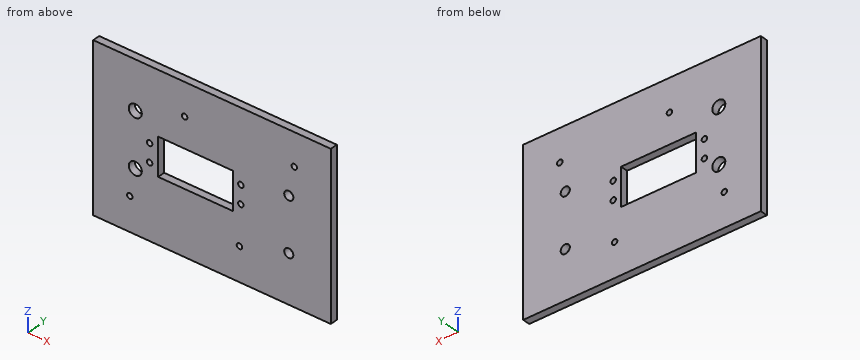
from build123d import *

# Parameters (mm, degrees)
SKETCH1_W           = 130
SKETCH1_H           = 90
BOSS_EXTRUDE1_DEPTH = 4
SKETCH7_R           = 3.65
SKETCH7_R_2         = 3.57
CUT_EXTRUDE5_DEPTH  = 10
SKETCH15_W          = 40.9
SKETCH15_H          = 20.7
CUT_EXTRUDE10_DEPTH = 5
SKETCH6_R           = 1.5
CUT_EXTRUDE4_DEPTH  = 4
SKETCH12_R          = 1.5
CUT_EXTRUDE8_DEPTH  = 5
SKETCH14_W          = 15.685038152
SKETCH14_H          = 44.965808151
SKETCH14_R          = 2.5
BOSS_EXTRUDE2_DEPTH = 4


with BuildPart() as part:
    # Sketch1 → Boss-Extrude1 (new body)
    with BuildSketch(Plane(origin=(0, 0, 0), x_dir=(1, 0, 0), z_dir=(0, 1, 0))):
        with Locations((-40, -6.672366697)):
            Rectangle(SKETCH1_W, SKETCH1_H)
    extrude(amount=BOSS_EXTRUDE1_DEPTH)

    # Sketch7 → Cut-Extrude5 (cut)
    with BuildSketch(Plane(origin=(0, 4, 0), x_dir=(1, 0, 0), z_dir=(0, 1, 0))):
        with Locations((2, 11.827633303)):
            Circle(SKETCH7_R)
        with Locations((2, -17.738049342)):
            Circle(SKETCH7_R)
        with Locations((-82, 4.393315947)):
            Circle(SKETCH7_R_2)
        with Locations((-82, -25.172366697)):
            Circle(SKETCH7_R_2)
    extrude(amount=-CUT_EXTRUDE5_DEPTH, mode=Mode.SUBTRACT)

    # Sketch15 → Cut-Extrude10 (cut, through all)
    with BuildSketch(Plane(origin=(0, 4, 0), x_dir=(1, 0, 0), z_dir=(0, 1, 0))):
        with Locations((-49, -7.030465848)):
            Rectangle(SKETCH15_W, SKETCH15_H)
    extrude(amount=-CUT_EXTRUDE10_DEPTH, mode=Mode.SUBTRACT)

    # Sketch6 → Cut-Extrude4 (cut)
    with BuildSketch(Plane.XZ):
        with Locations((-74.139435372, 12.030465848)):
            Circle(SKETCH6_R)
        with Locations((-24.239435372, 12.030465848)):
            Circle(SKETCH6_R)
        with Locations((-74.139435372, 2.030465848)):
            Circle(SKETCH6_R)
        with Locations((-24.239435372, 2.030465848)):
            Circle(SKETCH6_R)
    extrude(amount=-CUT_EXTRUDE4_DEPTH, mode=Mode.SUBTRACT)

    # Sketch12 → Cut-Extrude8 (cut, through all)
    with BuildSketch(Plane(origin=(0, 4, 0), x_dir=(1, 0, 0), z_dir=(0, 1, 0))):
        with Locations((-85, 19.819534152)):
            Circle(SKETCH12_R)
        with Locations((-25, 19.819534152)):
            Circle(SKETCH12_R)
        with Locations((-55, -33.880465848)):
            Circle(SKETCH12_R)
        with Locations((5, -33.880465848)):
            Circle(SKETCH12_R)
    extrude(amount=-CUT_EXTRUDE8_DEPTH, mode=Mode.SUBTRACT)

    # Sketch14 → Boss-Extrude2 (add, through all)
    with BuildSketch(Plane(origin=(0, 4, 0), x_dir=(1, 0, 0), z_dir=(0, 1, 0))):
        with Locations((2, -2.95520802)):
            Rectangle(SKETCH14_W, SKETCH14_H)
        with Locations((2, 11.827633303)):
            Circle(SKETCH14_R, mode=Mode.SUBTRACT)
        with Locations((2, -17.738049342)):
            Circle(SKETCH14_R, mode=Mode.SUBTRACT)
    extrude(amount=-BOSS_EXTRUDE2_DEPTH)


solid = part.part
Verification items for the finished model (mm, model axes). Coordinates: 2 decimals unless noted, no trailing zeros. Order: outer loops, then holes, each group sorted by start corner. A loop starts at its lowest first (then second) coordinate and runs counter-clockwise, first axis right, second up. Notation, with made-up numbers: M -34.5,-5.75 L -27.5,-5.75 A11 cw -27.5,9.25 Z; hole C -31.75,49.25 d11. An arc over 180 degrees is marked long. Write each question's results on one line, items separated by ' | '.
1) Section check C-C on x = 2. Record the cut outline in (y, z), plus the area to 3 significant figures.
Solved:
outline: M 0,-38.33 L 4,-38.33 L 4,-14.33 L 0,-14.33 Z; M 0,-9.33 L 4,-9.33 L 4,15.24 L 0,15.24 Z; M 0,20.24 L 4,20.24 L 4,51.67 L 0,51.67 Z | area: 320 mm²
2) Section check B-B on z = 7. Record the cut outline in (x, y), plus the area to 3 significant figures.
Solved:
outline: M -105,0 L -69.45,0 L -69.45,4 L -105,4 Z; M -28.55,0 L 25,0 L 25,4 L -28.55,4 Z | area: 356 mm²
3) Section check D-D on y = 1.6. Give the number of separate pieces and of enclosed holes in the cut face, plus the area to 3 significant figures.
Solved:
separate pieces: 1 | enclosed holes: 13 | area: 10,700 mm²
4) Scan lines: line 1 along Z through (x, y) = (-82, 1.8); line 2 along X through (y, z) = (1.9, 34); line 3 along Z through (x, y) = (-55, 2.65). Record each from-to range of solid material in increasing order. Write a range as [from, to].
Solved:
line 1: z = [-38.33, -7.96], [-0.82, 21.6], [28.74, 51.67] | line 2: x = [-105, -56.5], [-53.5, 3.5], [6.5, 25] | line 3: z = [-38.33, -3.32], [17.38, 32.38], [35.38, 51.67]
5) Section check A-A on x = -55. Record the cut outline in (y, z).
Solved:
outline: M 0,-38.33 L 4,-38.33 L 4,-3.32 L 0,-3.32 Z; M 0,17.38 L 4,17.38 L 4,32.38 L 0,32.38 Z; M 0,35.38 L 4,35.38 L 4,51.67 L 0,51.67 Z
6) Gauge pin test, flat ends, axial feed: pin 1 Ø4 at (x, z) = (5, 33.88) entering from +Y; pin 2 Ø1.8 at (x, z) = (-85, -19.82) entering from +Y. Record the tip position at first contact, or that the pin passes through.
Solved:
pin 1: stops at y = 4 | pin 2: passes through
